Check sheet for the modelled part. Datum: model origin and axes. Units: mm. Face numbers are marked on the shaded views. A direction names the side the tool comes from. Give positions to 0.01 mm unless a question says otherwise; leave off trailing zeros. Write each loop counter-clockwise with the first axis right and the second up, starting at its lowest first coordinate (ties: lowest second). Pieces come first, ordered by that corner, then holes. Notation, with made-up numbers: (37, 13.25) -> (42, 13.25) arc R29 ccw to (42, 46.25) -> close; hole circle Ø10 at (20.5, 14). An arc over 180 degrees is marked (long way). Return JSON: item names as keys, results as strings.
from build123d import *

# Parameters (mm, degrees)
SKETCH_R          = 8.5
SKETCH_R_2        = 1.5
PAD_DEPTH         = 3
SKETCH001_R       = 2
PAD001_DEPTH      = 3
PAD001_DEPTH_BACK = 20


with BuildPart() as part:
    # Sketch → Pad (new body)
    with BuildSketch(Plane.XY):
        Circle(SKETCH_R)
        Circle(SKETCH_R_2, mode=Mode.SUBTRACT)
    extrude(amount=PAD_DEPTH)

    # Sketch001 → Pad001 (new body, two sides)
    with BuildSketch(Plane(origin=(0, 0, 0), x_dir=(1, 0, 0), z_dir=(0, 0, -1))) as pad001_sk:
        with Locations((0, 6)):
            Circle(SKETCH001_R)
        with Locations((6, 0)):
            Circle(SKETCH001_R)
        with Locations((-6, 0)):
            Circle(SKETCH001_R)
        with Locations((0, -6)):
            Circle(SKETCH001_R)
    extrude(amount=PAD001_DEPTH)
    extrude(pad001_sk.sketch, amount=-PAD001_DEPTH_BACK)


solid = part.part
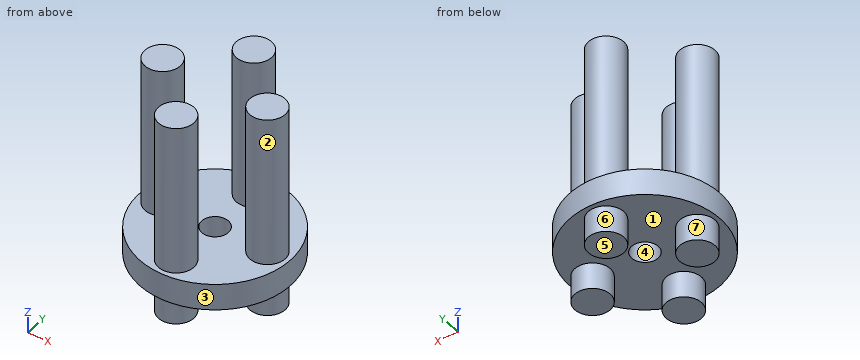
(1) Cross-section at D-D on x = -6. Enter the section's corners in (y, z).
Reply:
{"outline": "(-6.02, 0) -> (-2, 0) -> (-2, -3) -> (2, -3) -> (2, 0) -> (6.02, 0) -> (6.02, 3) -> (2, 3) -> (2, 20) -> (-2, 20) -> (-2, 3) -> (-6.02, 3) -> close"}
(2) Thickness scan on L1, parallel to Y at x = 0, z = 1.4; L2, parallel to Y at x = 1, z = 2.5; L3, parallel to Z at x = -3, y = 1.25. Record the ranges inside material, lowest first.
Reply:
{"L1": "-8.5 to -1.5, 1.5 to 8.5", "L2": "-8.44 to -1.12, 1.12 to 8.44", "L3": "0 to 3"}
(3) Release check for a two-part mould opening along X. For the marked faces 4, 5, 6 and 7 record: pulls with the +X half, pulls with the -X half, needs draft (parallel to the pull), parting line crosses it, or undercut.
Reply:
{"face 4": "undercut", "face 5": "needs draft", "face 6": "parting line crosses it", "face 7": "undercut"}
(4) Depth check by flat-ended pin: pin 1 Ø1 at (x, y) = (-1.5, 3.5) entering from +Z; pin 2 Ø4 at (x, z) = (-3, 1) entering from -Y; pin 3 Ø6 at (x, y) = (1.5, -2) entering from +Z; pin 4 Ø5 at (x, z) = (1, 11) entering from +Y. Enter the tip coordinate at first touch or a pass-through.
Reply:
{"pin 1": "z = 3", "pin 2": "y = -8.44", "pin 3": "z = 20", "pin 4": "y = 8"}
(5) Cross-section at C-C on z = 13.5. Enter the section's corners in (x, y).
Reply:
{"outline": "circle Ø4 at (-6, 0); circle Ø4 at (0, -6); circle Ø4 at (0, 6); circle Ø4 at (6, 0)"}
(6) Cross-section at A-A on y = 0. Enter the section's corners in (x, z).
Reply:
{"outline": "(-8.5, 0) -> (-8, 0) -> (-8, -3) -> (-4, -3) -> (-4, 0) -> (-1.5, 0) -> (-1.5, 3) -> (-4, 3) -> (-4, 20) -> (-8, 20) -> (-8, 3) -> (-8.5, 3) -> close; (1.5, 0) -> (4, 0) -> (4, -3) -> (8, -3) -> (8, 0) -> (8.5, 0) -> (8.5, 3) -> (8, 3) -> (8, 20) -> (4, 20) -> (4, 3) -> (1.5, 3) -> close"}
(7) Set-up check for the marked faces 1, 2 and 3: record each of +Z, -Z, +X, -X, +Y, -Y from which the full face is reachable in a straight line by a thin tool's end or side.
Reply:
{"face 1": "-Z", "face 2": "+Z", "face 3": "+Z, -Z"}
